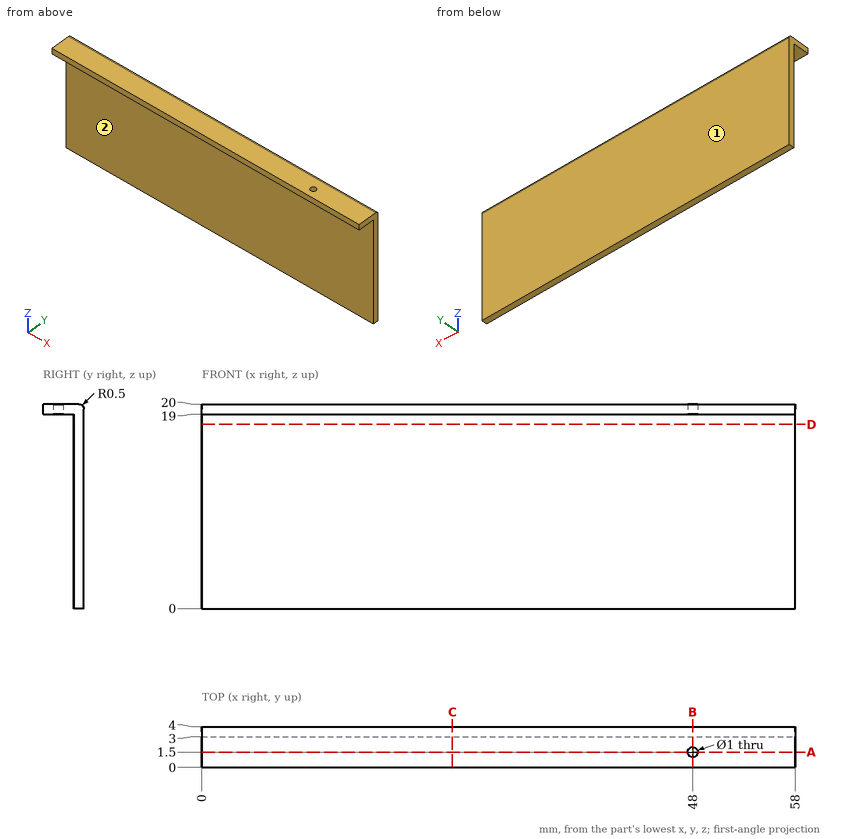
Part print with two shaded views. Sizes in mm from the minimum x, y, z corner. A direction names the side the tool comes from. Round coordinates to 2 decimals unless told otherwise and drop trailing zeros. Write each loop counter-clockwise with the first axis right and the second up, starting at its lowest first coordinate (ties: lowest second). Pieces come first, ordered by that corner, then holes. Notation, with made-up numbers: M 21.5,6 L 56.5,6 A27 cw 56.5,45 Z; hole C 3.25,-7 d7. An arc over 180 degrees is marked long. Put each result on its own line as item: value. Start each with the question number.
1) Drill centre lines: probe 1 along Y at (x, z) = (48, 19.6); probe 2 along Z at (x, y) = (42, 1.6); probe 3 along Y at (x, z) = (16, 3.25). Where is each one in solid material? Low to high. Write a range as [from, to].
2) Pin check, flat tips, straight feed: pin 1 Ø1.5 at (x, y) = (30, 1.5) entering from -Z; pin 2 Ø2 at (x, z) = (26.5, 5.5) entering from -Y. Stop position of each tip, or through.
3) Saw through at C-C, the plane x = 24.5. Write the cut outline in (y, z).
4) 3-axis set-ups, long thin cutter, end or side, ignore diameter. For the marked faces 1 and 2: which of +Z, -Z, +X, -X, +Y, -Y reach the whole face in a straight line?
5) Saw through at B-B, the plane x = 48. Write the cut outline in (y, z), and give its area (3 significant figures).
6) Saw through at D-D, the plane z = 18. Write the cut outline in (x, y).
7) Saw through at A-A, the plane y = 1.5. Write the cut outline in (x, z), and give its area (3 significant figures).
Resolved:
1. probe 1: [0, 1], [2, 3.99]
1. probe 2: [19, 20]
1. probe 3: [3, 4]
2. pin 1: z = 19
2. pin 2: y = 3
3. outline: M 0,19 L 3,19 L 3,0 L 4,0 L 4,19.5 A0.5 ccw 3.5,20 L 0,20 Z
4. face 1: +Z, -Z, +X, -X, +Y
4. face 2: -Z, +X, -X, -Y
5. outline: M 0,19 L 1,19 L 1,20 L 0,20 Z; M 2,19 L 3,19 L 3,0 L 4,0 L 4,19.5 A0.5 ccw 3.5,20 L 2,20 Z
5. area: 21.9 mm²
6. outline: M 0,3 L 58,3 L 58,4 L 0,4 Z
7. outline: M 0,19 L 47.5,19 L 47.5,20 L 0,20 Z; M 48.5,19 L 58,19 L 58,20 L 48.5,20 Z
7. area: 57.0 mm²
